Here's how the part is built. I have some questions about the finished solid (model axes, mm). Coordinates: 2 decimals unless noted, no trailing zeros. Write each loop counter-clockwise with the first axis right and the second up, starting at its lowest first coordinate (ties: lowest second). Pieces come first, ordered by that corner, then holes. Notation, with made-up numbers: M 76,-14 L 101,-14 A19 cw 101,18 Z; hole C 65,16.5 d4. An arc over 180 degrees is marked long. Use one line per item in the form item = value. Start each with the question number.
1. I want a section at A-A, the plane y = -167. List the corners of the cut face in (x, z) for me, plus the area to 3 significant figures.
2. I'm going to push a flat-ended pin straight in: pin 1 Ø0.5 at (x, z) = (440.5, -0.5) entering from -Y. Where does the tip first touch, or does it pass through?
3. I want a section at B-B, the plane z = -0.3. Count the separate pieces of the cut face and the enclosed holes in it, plus the area to 3 significant figures.
4. Please list where these lines run through material, in increasing order: line 1 along X through (y, z) = (294.45, -0.45); line 2 along Y through (x, z) = (419, -0.4) (3 decimals); line 3 along Y through (x, z) = (443, -0.15). Write a range as [from, to].
from build123d import *

# Parameters (mm, degrees)
SKETCH1_W            = 856
SKETCH1_H            = 606.9
BASE_FLANGE1_DEPTH   = 1
M5_CLEARANCE_HOLE1_D = 5.5
M8_CLEARANCE_HOLE1_D = 9
LPATTERN1_COUNT      = 5
LPATTERN1_PITCH      = 192.5
FILLET1_R            = 10
M4_CLEARANCE_HOLE1_D = 4.5
SKETCH8_R            = 4.25
BOSS_EXTRUDE1_DEPTH  = 1
FILLET2_R            = 10


# Sheet-metal steps are written as plain solids
with BuildPart() as part:
    # Sketch1 → Base-Flange1 (new body)
    with BuildSketch(Plane.XY):
        Rectangle(SKETCH1_W, SKETCH1_H)
    extrude(amount=-BASE_FLANGE1_DEPTH)

    # M5 Clearance Hole1 (through all)
    with Locations(Plane(origin=(0, 0, -1), x_dir=(-1, 0, 0), z_dir=(0, 0, -1))):
        with Locations((-419, -282.45), (-419, -149.225), (-419, -16), (-419, 117.225), (-419, 250.45), (-408, 294.45), (-204, 294.45), (0, 294.45), (204, 294.45), (408, 294.45), (419, 250.45), (419, 117.225), (419, -16), (419, -149.225), (419, -282.45)):
            Hole(M5_CLEARANCE_HOLE1_D / 2)

    # M8 Clearance Hole1 (through all)
    with Locations(Plane.XY):
        with Locations((-385, -283.45)):
            m8_clearance_hole1 = Hole(M8_CLEARANCE_HOLE1_D / 2)

    # LPattern1: M8 Clearance Hole1 ×5
    with Locations(*[(i * LPATTERN1_PITCH, 0, 0) for i in range(1, LPATTERN1_COUNT)]):
        add(m8_clearance_hole1, mode=Mode.SUBTRACT)

    # Fillet1
    fillet1_edges = [part.edges().sort_by_distance(p)[0] for p in [
        (428, -303.45, -0.5),
        (-428, -303.45, -0.5),
        (-428, 303.45, -0.5),
        (428, 303.45, -0.5),
    ]]
    fillet(fillet1_edges, radius=FILLET1_R)

    # M4 Clearance Hole1 (through all)
    with Locations(Plane.XY):
        with Locations((267, -283.45), (303, -283.45)):
            Hole(M4_CLEARANCE_HOLE1_D / 2)

    # Sketch8 → Boss-Extrude1 (add)
    with BuildSketch(Plane.XY):
        with BuildLine():
            Line((-428, 53.55), (-443, 53.55))
            ThreePointArc((-443, 53.55), (-460.67766953, 46.22766953), (-468, 28.55))
            Line((-468, 28.55), (-468, -88.45))
            ThreePointArc((-468, -88.45), (-460.67766953, -106.12766953), (-443, -113.45))
            Line((-443, -113.45), (-428, -113.45))
            Line((-428, -113.45), (-428, 53.55))
        make_face()
        with Locations((-443, 28.55)):
            Circle(SKETCH8_R, mode=Mode.SUBTRACT)
        with Locations((-443, -88.45)):
            Circle(SKETCH8_R, mode=Mode.SUBTRACT)
    boss_extrude1 = extrude(amount=-BOSS_EXTRUDE1_DEPTH)

    # Mirror3: Boss-Extrude1 across plane
    add(boss_extrude1.mirror(Plane(origin=(0, 0, 0), x_dir=(0, 0, 1), z_dir=(1, 0, 0))))

    # Fillet2
    fillet2_edges = [part.edges().sort_by_distance(p)[0] for p in [
        (-428, 53.55, -0.5),
        (-428, -113.45, -0.5),
        (428, -113.45, -0.5),
        (428, 53.55, -0.5),
    ]]
    fillet(fillet2_edges, radius=FILLET2_R)


solid = part.part
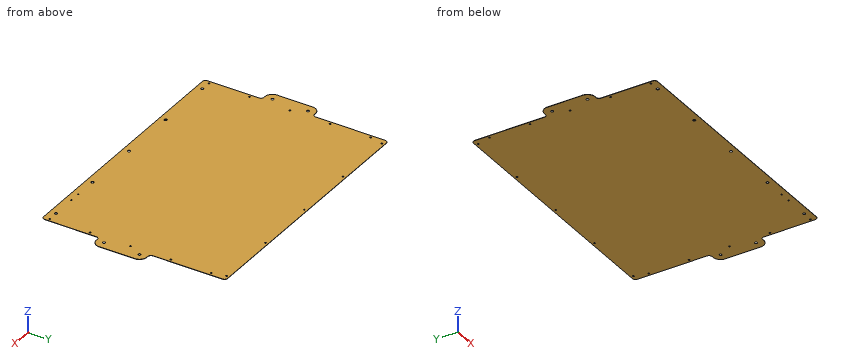
Answer list:
q1.outline = M -428,-1 L 428,-1 L 428,0 L -428,0 Z
q1.area = 856 mm²
q2.pin_1 = -113.45
q3.separate_pieces = 1
q3.enclosed_holes = 26
q3.area = 531,000 mm²
q4.line_1 = [-427.95, -410.75], [-405.25, -206.75], [-201.25, -2.75], [2.75, 201.25], [206.75, 405.25], [410.75, 427.95]
q4.line_2 = [-303.4, -285.2], [-279.7, -151.975], [-146.475, -18.75], [-13.25, 114.475], [119.975, 247.7], [253.2, 303.4]
q4.line_3 = [-113.45, -92.7], [-84.2, 24.3], [32.8, 53.55]
